Here's how the part is built. I have some questions about the finished solid (model axes, mm). A direction names the side the tool comes from. Coordinates: 2 decimals unless noted, no trailing zeros. Write each loop counter-clockwise with the first axis right and the second up, starting at its lowest first coordinate (ties: lowest second). Pieces come first, ordered by that corner, then holes.
```python
from build123d import *
from build123d.topology import SkipClean

# Parameters (mm, degrees)
BOSS_EXTRUDE1_DEPTH  = 6
SKETCH2_W            = 6
SKETCH2_H            = 6
SKETCH2_R            = 1.525
BOSS_EXTRUDE2_DEPTH  = 3.75
FILLET1_R            = 3
SKETCH4_W            = 33.355842528
SKETCH4_H            = 6
BOSS_EXTRUDE3_DEPTH  = 3
BOSS_EXTRUDE4_DEPTH  = 33.355842528
BOSS_EXTRUDE5_START  = -6.75
SKETCH7_R            = 1.525
BOSS_EXTRUDE5_DEPTH  = 12
SKETCH8_W            = 6
SKETCH8_H            = 5.25
BOSS_EXTRUDE6_DEPTH  = 1.433789
BOSS_EXTRUDE7_REACH  = 51.468
SKETCH11_W           = 6
SKETCH11_H           = 3
MIRROR1_START        = -14.24613882
MIRROR1_OUTLINE_R    = 1.525
MIRROR1_DEPTH        = 12
SKETCH13_W           = 6
SKETCH13_H           = 5.25
BOSS_EXTRUDE8_DEPTH  = 1.434493
BOSS_EXTRUDE9_REACH  = 51.468
SKETCH14_W           = 6
SKETCH14_H           = 3
CHAMFER1_SIZE        = 2
SKETCH15_W           = 7.967920834
SKETCH15_H           = 6.3175
CUT_EXTRUDE1_DEPTH   = 6.25
BOSS_EXTRUDE10_DEPTH = 6


# Read off the part's stored shape, not the designer's step: Mirror1
# Some blends are built 0.0001 mm under size
with BuildPart() as part:
    # Sketch1 → Boss-Extrude1 (new body)
    with BuildSketch(Plane(origin=(0, 0, 0.755649514), x_dir=(-1, 0, 0), z_dir=(0, 0, -1))):
        Polygon((31.089725273, -5.24613882), (30.270792245, -7.49613882), (29.667061326, -7.49613882), (29.667061326, -11.24613882), (70.667061326, -11.24613882), (70.827061326, -11.24613882), (70.827061326, -7.49613882), (70.667061326, -7.49613882), (70.222625956, -7.49613882), (69.403692929, -5.24613882), (68.788837073, -5.24613882), (67.969904045, -7.49613882), (67.081033306, -7.49613882), (66.262100279, -5.24613882), (65.647244423, -5.24613882), (64.828311395, -7.49613882), (63.939440656, -7.49613882), (63.120507629, -5.24613882), (62.505651773, -5.24613882), (61.686718745, -7.49613882), (60.797848006, -7.49613882), (59.978914979, -5.24613882), (59.364059123, -5.24613882), (58.545126095, -7.49613882), (57.656255356, -7.49613882), (56.837322329, -5.24613882), (56.222466473, -5.24613882), (55.403533445, -7.49613882), (54.514662706, -7.49613882), (53.695729679, -5.24613882), (53.080873823, -5.24613882), (52.261940795, -7.49613882), (51.373070056, -7.49613882), (50.554137029, -5.24613882), (49.939281173, -5.24613882), (49.120348145, -7.49613882), (48.231477406, -7.49613882), (47.412544379, -5.24613882), (46.797688523, -5.24613882), (45.978755495, -7.49613882), (45.089884756, -7.49613882), (44.270951729, -5.24613882), (43.656095873, -5.24613882), (42.837162845, -7.49613882), (41.948292106, -7.49613882), (41.129359079, -5.24613882), (40.514503223, -5.24613882), (39.695570195, -7.49613882), (38.806699456, -7.49613882), (37.987766429, -5.24613882), (37.372910573, -5.24613882), (36.553977545, -7.49613882), (35.665106806, -7.49613882), (34.846173779, -5.24613882), (34.231317923, -5.24613882), (33.412384895, -7.49613882), (32.523514156, -7.49613882), (31.704581129, -5.24613882), align=None)
    extrude(amount=-BOSS_EXTRUDE1_DEPTH)

    # Sketch2 → Boss-Extrude2 (add)
    # profile 1 of 2: a face of its own
    with BuildSketch(Plane.XZ.offset(11.24613882)):
        with Locations((-73.827061326, 3.755649514)):
            Rectangle(SKETCH2_W, SKETCH2_H)
        with Locations(Location((-73.827061326, 3.755649514, 0), (0, 0, 270))):
            Circle(SKETCH2_R, mode=Mode.SUBTRACT)
    # profile 2 of 2: a face of its own
    with BuildSketch(Plane.XZ.offset(11.24613882)):
        with Locations((-26.667061326, 3.755649514)):
            Rectangle(SKETCH2_W, SKETCH2_H)
        with Locations(Location((-26.667061326, 3.755649514, 0), (0, 0, 270))):
            Circle(SKETCH2_R, mode=Mode.SUBTRACT)
    extrude(amount=-BOSS_EXTRUDE2_DEPTH)

    # Fillet1
    fillet1_edges = [part.edges().sort_by_distance(p)[0] for p in [
        (-23.667061326, -9.37113882, 0.755649514),
        (-23.667061326, -9.37113882, 6.755649514),
        (-76.827061326, -9.37113882, 6.755649514),
        (-76.827061326, -9.37113882, 0.755649514),
    ]]
    fillet(fillet1_edges, radius=FILLET1_R - 0.0001)  # a hair under: the kernel refuses the full size

    # Sketch4 → Boss-Extrude3 (add)
    with BuildSketch(Plane.XZ.offset(11.24613882)):
        with Locations((-50.247061326, 3.755649514)):
            Rectangle(SKETCH4_W, SKETCH4_H)
    extrude(amount=BOSS_EXTRUDE3_DEPTH)

    # Sketch5 → Boss-Extrude4 (add)
    with BuildSketch(Plane.ZY.offset(66.92498259)):
        Polygon((0.755649514, -11.24613882), (-1.244350486, -13.24613882), (-1.244350486, -14.24613882), (0.755649514, -14.24613882), align=None)
        Polygon((8.755649514, -13.24613882), (8.755649514, -14.24613882), (6.755649514, -14.24613882), (6.755649514, -11.24613882), align=None)
    extrude(amount=-BOSS_EXTRUDE4_DEPTH)

    # Sketch7 → Boss-Extrude5 (add)
    with BuildSketch(Plane(origin=(0, -7.49613882, 0), x_dir=(1, 0, 0), z_dir=(0, 1, 0)).offset(BOSS_EXTRUDE5_START)):
        with BuildLine():
            Line((-26.667061326, -0.755649514), (-30.270792245, -0.755649514))
            Line((-30.270792245, -0.755649514), (-30.270792245, -6.755649514))
            Line((-30.270792245, -6.755649514), (-26.667061326, -6.755649514))
            ThreePointArc((-26.667061326, -6.755649514), (-24.545740982, -5.876969858), (-23.667061326, -3.755649514))
            ThreePointArc((-23.667061326, -3.755649514), (-24.545740982, -1.634329171), (-26.667061326, -0.755649514))
        make_face()
        with Locations(Location((-26.667061326, -3.755649514, 0), (0, 0, 270))):
            Circle(SKETCH7_R, mode=Mode.SUBTRACT)
    extrude(amount=BOSS_EXTRUDE5_DEPTH)

    # Sketch8 → Boss-Extrude6 (add)
    with BuildSketch(Plane.ZY.offset(30.270792245)):
        with Locations((3.755649514, -4.87113882)):
            Rectangle(SKETCH8_W, SKETCH8_H)
    extrude(amount=BOSS_EXTRUDE6_DEPTH)

    # Sketch11 → Boss-Extrude7 (add, up to next)
    with BuildSketch(Plane.ZY.offset(30.270792245), mode=Mode.PRIVATE) as boss_extrude7_sk1:
        with Locations((3.755649514, -12.74613882)):
            Rectangle(SKETCH11_W, SKETCH11_H)
    boss_extrude7_tool1 = extrude(boss_extrude7_sk1.sketch, amount=BOSS_EXTRUDE7_REACH, mode=Mode.PRIVATE) - part.part
    add(boss_extrude7_tool1.solids().sort_by_distance((-30.270792, -12.746139, 3.75565))[0])

    # Mirror1 outline → Mirror1 (add)
    with SkipClean():  # the faces are left unmerged after this step: merging them gives an invalid solid
        with BuildSketch(Plane(origin=(0, 0, 0), x_dir=(1, 0, 0), z_dir=(0, 1, 0)).offset(MIRROR1_START)):
            with BuildLine():
                ThreePointArc((-73.827061326, -0.755649514), (-76.827061326, -3.755649514), (-73.827061326, -6.755649514))
                Line((-73.827061326, -6.755649514), (-70.223330406, -6.755649514))
                Line((-70.223330406, -6.755649514), (-70.223330406, -0.755649514))
                Line((-70.223330406, -0.755649514), (-73.827061326, -0.755649514))
            make_face()
            with Locations((-73.827061326, -3.755649514)):
                Circle(MIRROR1_OUTLINE_R, mode=Mode.SUBTRACT)
        extrude(amount=MIRROR1_DEPTH)

    # Sketch13 → Boss-Extrude8 (add)
    with SkipClean():  # the faces are left unmerged after this step: merging them gives an invalid solid
        with BuildSketch(Plane(origin=(-70.223330406, 0, 0), x_dir=(0, 0, -1), z_dir=(1, 0, 0))):
            with Locations((-3.755649514, -4.87113882)):
                Rectangle(SKETCH13_W, SKETCH13_H)
        extrude(amount=BOSS_EXTRUDE8_DEPTH)

    # Sketch14 → Boss-Extrude9 (add, up to next)
    with BuildSketch(Plane(origin=(-70.223330406, 0, 0), x_dir=(0, 0, -1), z_dir=(1, 0, 0)), mode=Mode.PRIVATE) as boss_extrude9_sk1:
        with Locations((-3.755649514, -12.74613882)):
            Rectangle(SKETCH14_W, SKETCH14_H)
    boss_extrude9_tool1 = extrude(boss_extrude9_sk1.sketch, amount=BOSS_EXTRUDE9_REACH, mode=Mode.PRIVATE) - part.part
    add(boss_extrude9_tool1.solids().sort_by_distance((-70.22333, -12.746139, 3.75565))[0])

    # Chamfer1
    # the kernel refuses this chamfer: 2 mm, written as the material it takes off along each edge
    with BuildSketch(Plane(origin=(-31.704581245, -2.24613882, 11.89901549), x_dir=(0.9996219169112968, 0.027495876610586296, 0), z_dir=(0, 0, -1))) as chamfer1_piece_1:
        Polygon((CHAMFER1_SIZE * 0.999621916911, CHAMFER1_SIZE * 0.0274958766106), (-CHAMFER1_SIZE * 0.0274958766106, CHAMFER1_SIZE * 0.999621916911), (0, 0), align=None)
    extrude(amount=16.286731952, mode=Mode.SUBTRACT)
    with BuildSketch(Plane(origin=(-68.788837406, -2.24613882, -4.387716461), x_dir=(0.027495876610589064, -0.9996219169112965, 0), z_dir=(0, 0, 1))) as chamfer1_piece_2:
        Polygon((CHAMFER1_SIZE * 0.999621916911, -CHAMFER1_SIZE * 0.0274958766106), (-CHAMFER1_SIZE * 0.0274958766106, -CHAMFER1_SIZE * 0.999621916911), (0, 0), align=None)
    extrude(amount=16.286731952, mode=Mode.SUBTRACT)

    # Sketch15 → Cut-Extrude1 (cut)
    with BuildSketch(Plane(origin=(0, 0, 0.755649514), x_dir=(-1, 0, 0), z_dir=(0, 0, -1))):
        with Locations((25.720620712, -8.08738882)):
            Rectangle(SKETCH15_W, SKETCH15_H)
    cut_extrude1 = extrude(amount=-CUT_EXTRUDE1_DEPTH, mode=Mode.SUBTRACT)

    # Mirror2: Cut-Extrude1 across plane
    add(cut_extrude1.mirror(Plane(origin=(-50.247061326, 0, 0), x_dir=(0, 0, 1), z_dir=(1, 0, 0))), mode=Mode.SUBTRACT)

    # Sketch16 → Boss-Extrude10 (add)
    with BuildSketch(Plane(origin=(0, 0, 0.755649514), x_dir=(-1, 0, 0), z_dir=(0, 0, -1))):
        Polygon((67.969904045, -7.49613882), (68.788837073, -4.24613882), (68.788837073, -7.702493067), align=None)
        Polygon((31.704581129, -4.24613882), (32.523514156, -7.49613882), (31.704581129, -7.702493067), align=None)
    extrude(amount=-BOSS_EXTRUDE10_DEPTH)


solid = part.part
```
1) We'd pull the mould along X, two halves only. Please class faces 1 (the face through (-48.7, -7.496, 3.7)), 2 (the face through (-29.705, -8, 4)), 3 (the face through (-76.826, -12.767, 3.69)), 4 (the face through (-51, -8, 0.756)): pulls with the +X half, pulls with the -X half, needs draft (parallel to the pull), parting line crosses it, or undercut.
Values follow:
face 1: undercut
face 2: pulls with the +X half
face 3: pulls with the -X half
face 4: needs draft
2) I need wall thicknesses on probe 1 along X at (y, z) = (-4.75, 2.75); probe 2 along X at (y, z) = (-4.5, 4.25); probe 3 along X at (y, z) = (-11, 6.5). Which ranges of each line are inside material? Lowest first, please.
Values follow:
probe 1: x = -76.65 to -74.97, -72.68 to -68.66, -31.83 to -27.81, -25.52 to -23.84
probe 2: x = -76.79 to -75.27, -72.38 to -68.72, -31.77 to -28.11, -25.22 to -23.71
probe 3: x = -70.79 to -29.7
3) On a 3-axis mill with a long thin cutter (end or side, diameter ignored), from which of +Z, -Z, +X, -X, +Y, -Y can I reach the whole of each face in a straight line? I mean faces 5 (the face through (-27, -2.246, 2)), 6 (the face through (-49.536, -6.355, 3.714)). Say none if no direction works.
Values follow:
face 5: +Z, -Z, +X, -X, +Y
face 6: +Z, -Z, +Y
4) Imagine slicing it at C-C on z = -0.5. Please give me the cut outline in (x, y), then the cut area to 3 significant figures.
Values follow:
outline: (-66.92, -14.25) - (-33.57, -14.25) - (-33.57, -12.5) - (-66.92, -12.5) - close
area: 58.2 mm2
5) Will these pins go through, and if not, where does the flat tip stop? pin 1 (1 mm diameter, centred on y = -13, z = -0.5, fed in from -X) (3 decimals); pin 2 (0.5 mm diameter, centred on x = -56.5, z = 2.5, fed in from +Y); pin 3 (3 mm diameter, centred on y = -7, z = 4, fed in from +X).
Values follow:
pin 1: stops at x = -66.925
pin 2: stops at y = -5.25
pin 3: stops at x = -29.7
6) Imagine slicing it at B-B on y = -12.25. Please give me the cut outline in (x, z) (3 decimals).
Values follow:
outline: (-73.827, 0.756) - (-66.925, 0.756) - (-66.925, -0.248) - (-33.569, -0.248) - (-33.569, 0.756) - (-26.667, 0.756) arc R3 ccw to (-26.667, 6.756) - (-33.569, 6.756) - (-33.569, 7.76) - (-66.925, 7.76) - (-66.925, 6.756) - (-73.827, 6.756) arc R3 ccw to start; hole circle Ø3.05 at (-73.827, 3.756); hole circle Ø3.05 at (-26.667, 3.756)
7) Imagine slicing it at A-A on y = -3.25. Please give me the cut outline in (x, z) (3 decimals).
Values follow:
outline: (-73.827, 0.756) - (-69.785, 0.756) - (-69.785, 6.756) - (-73.827, 6.756) arc R3 ccw to start; (-30.708, 0.756) - (-26.667, 0.756) arc R3 ccw to (-26.667, 6.756) - (-30.708, 6.756) - close; hole circle Ø3.05 at (-73.827, 3.756); hole circle Ø3.05 at (-26.667, 3.756)
